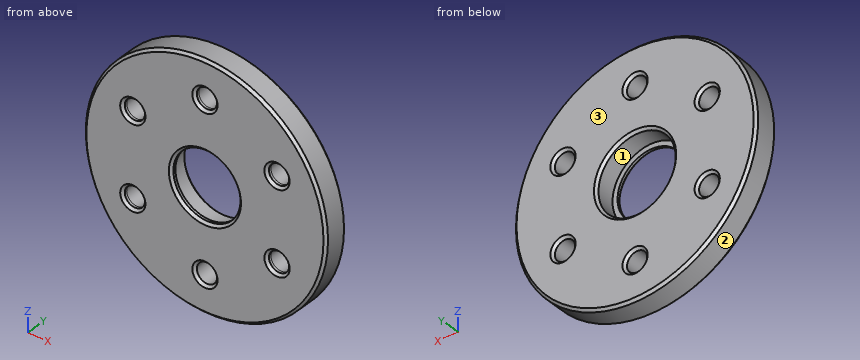
from build123d import *

# Parameters (mm, degrees)
SKETCH1_R           = 24
SKETCH1_R_2         = 7.65
BOSS_EXTRUDE1_DEPTH = 4
SKETCH2_R           = 2
CUT_EXTRUDE1_DEPTH  = 5
CIRPATTERN2_COUNT   = 6
SKETCH3_R           = 24
SKETCH3_R_2         = 6.65
SKETCH3_R_3         = 2
BOSS_EXTRUDE2_DEPTH = 1
CHAMFER1_SIZE       = 0.5


with BuildPart() as part:
    # Sketch1 → Boss-Extrude1 (new body)
    with BuildSketch(Plane(origin=(0, 0, 0), x_dir=(1, 0, 0), z_dir=(0, 1, 0))):
        Circle(SKETCH1_R)
        Circle(SKETCH1_R_2, mode=Mode.SUBTRACT)
    extrude(amount=BOSS_EXTRUDE1_DEPTH)

    # Sketch2 → Cut-Extrude1 (cut, through all)
    with BuildSketch(Plane(origin=(0, 4, 0), x_dir=(1, 0, 0), z_dir=(0, 1, 0))):
        with Locations((0, 16.5)):
            Circle(SKETCH2_R)
    cut_extrude1 = extrude(amount=-CUT_EXTRUDE1_DEPTH, mode=Mode.SUBTRACT)

    # CirPattern2: Cut-Extrude1 ×6 about axis
    cirpattern2_axis = Axis((0, 0, 0), (0, 1, 0))
    for i in range(1, CIRPATTERN2_COUNT):
        add(cut_extrude1.rotate(cirpattern2_axis, i * 360 / CIRPATTERN2_COUNT), mode=Mode.SUBTRACT)

    # Sketch3 → Boss-Extrude2 (add)
    with BuildSketch(Plane(origin=(0, 0, 0), x_dir=(1, 0, 0), z_dir=(0, 1, 0))):
        Circle(SKETCH3_R)
        Circle(SKETCH3_R_2, mode=Mode.SUBTRACT)
        with Locations((-14.289419, -8.25)):
            Circle(SKETCH3_R_3, mode=Mode.SUBTRACT)
        with Locations((0, -16.5)):
            Circle(SKETCH3_R_3, mode=Mode.SUBTRACT)
        with Locations((14.289419, -8.25)):
            Circle(SKETCH3_R_3, mode=Mode.SUBTRACT)
        with Locations((14.289419, 8.25)):
            Circle(SKETCH3_R_3, mode=Mode.SUBTRACT)
        with Locations((0, 16.5)):
            Circle(SKETCH3_R_3, mode=Mode.SUBTRACT)
        with Locations((-14.289419, 8.25)):
            Circle(SKETCH3_R_3, mode=Mode.SUBTRACT)
    extrude(amount=-BOSS_EXTRUDE2_DEPTH)

    # Chamfer1
    chamfer1_edges = [part.edges().sort_by_distance(p)[0] for p in [
        (-2, 4, -16.5),
        (13.289419, 4, -9.982051),
        (15.289419, 4, 6.517949),
        (2, 4, 16.5),
        (-13.289419, 4, 9.982051),
        (-15.289419, 4, -6.517949),
        (-24, -1, 0),
        (-16.289419, -1, -8.25),
        (-2, -1, -16.5),
        (12.289419, -1, -8.25),
        (12.289419, -1, 8.25),
        (-2, -1, 16.5),
        (-6.65, -1, 0),
        (-16.289419, -1, 8.25),
        (-24, 4, 0),
        (-7.65, 4, 0),
    ]]
    chamfer(chamfer1_edges, length=CHAMFER1_SIZE)


solid = part.part
For this review, take the finished solid that the model builds, in its own axes (mm). Face numbers are marked on the shaded views. Give positions to 0.01 mm unless a question says otherwise; leave off trailing zeros. Write each loop counter-clockwise with the first axis right and the second up, starting at its lowest first coordinate (ties: lowest second). Pieces come first, ordered by that corner, then holes. Notation, with made-up numbers: (72, -23.5) -> (83, -23.5) arc R19 cw to (83, -11.5) -> close; hole circle Ø11 at (75, 52). An arc over 180 degrees is marked (long way). Use CSV: the item, a comma, the result in double quotes.
Q1. Take a section at B-B, the plane x = 0. State how many separate pieces and enclosed holes the cut face has, then the cut area to 4 significant figures.
Conclusion:
separate pieces,"4"
enclosed holes,"0"
area,"123.5 mm2"
Q2. Take a section at A-A, the plane z = 0. Write out the cut boundary in (x, y).
Conclusion:
outline,"(-24, -0.5) -> (-23.5, -1) -> (-7.15, -1) -> (-6.65, -0.5) -> (-6.65, 0) -> (-7.65, 0) -> (-7.65, 3.5) -> (-8.15, 4) -> (-23.5, 4) -> (-24, 3.5) -> close; (6.65, -0.5) -> (7.15, -1) -> (23.5, -1) -> (24, -0.5) -> (24, 3.5) -> (23.5, 4) -> (8.15, 4) -> (7.65, 3.5) -> (7.65, 0) -> (6.65, 0) -> close"
Q3. To check wall thickness, follow probe 1 along Z at (x, y) = (0, 1.7); probe 2 along X at (y, z) = (3.45, -8); probe 3 along X at (y, z) = (-0.3, 8.25). State the ranges of each line that lie inside material, in increasing order. Write a range as [from, to].
Conclusion:
probe 1,"[-24, -18.5], [-14.5, -7.65], [7.65, 14.5], [18.5, 24]"
probe 2,"[-22.63, -16.27], [-12.31, 12.31], [16.27, 22.63]"
probe 3,"[-22.54, -16.29], [-12.29, 12.29], [16.29, 22.54]"
Q4. Mouldability with a two-part tool opening along Z and no side actions: class the marked faces 1, 2 and 3 as pulls with the +Z half, pulls with the -Z half, needs draft (parallel to the pull), parting line crosses it, or undercut.
Conclusion:
face 1,"undercut"
face 2,"parting line crosses it"
face 3,"needs draft"
Q5. For P1, Ø3, axis at y = 1.5, z = 18, coming from the -X side; P2, Ø3, axis at y = -0.5, z = -8.5, coming from the +X side; P3, Ø1.5, axis at x = 17.5, y = 2.5, coming from the -Z side, all flat-tipped, find the tip position at first contact; note any pin that passes through.
Conclusion:
P1,"x = -17.43"
P2,"x = 22.96"
P3,"z = -17.19"
